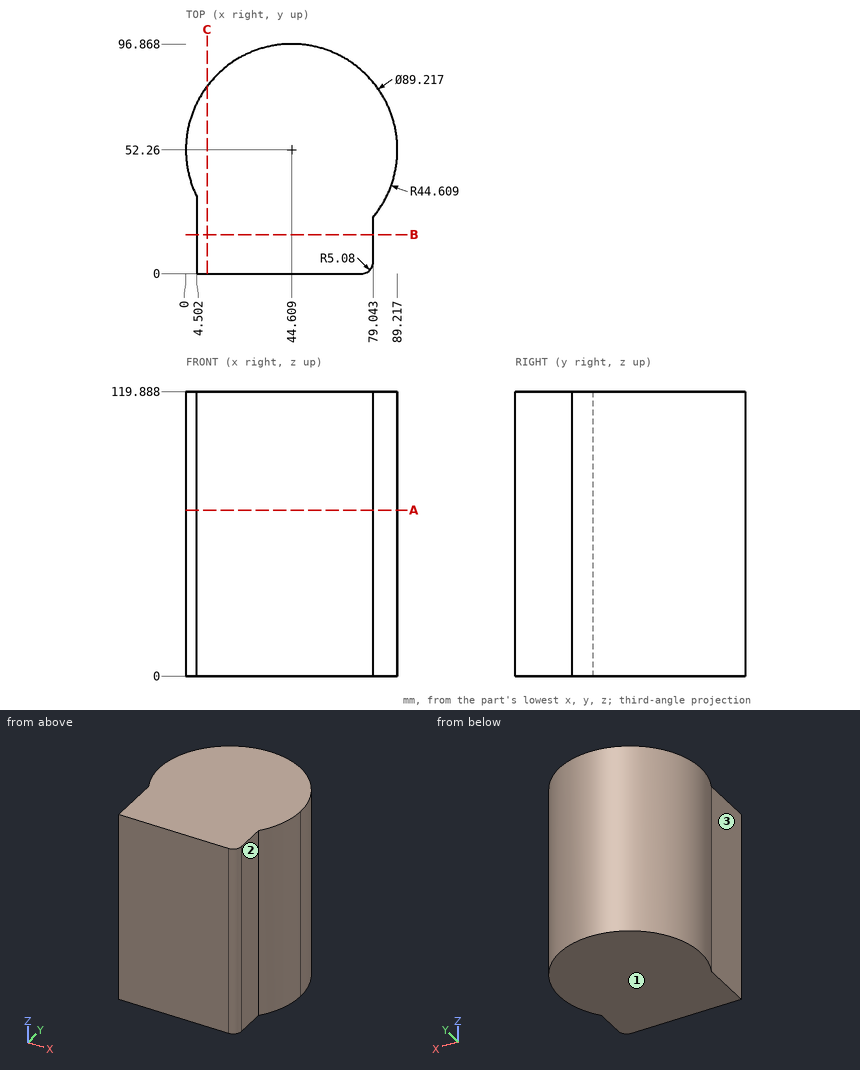
Input: dimensioned drawing with shaded views. Units: mm. Origin: part minimum x, y, z. A direction names the side the tool comes from. Give positions to 0.01 mm unless a question says otherwise; leave off trailing zeros. Order: outer loops, then holes, each group sorted by start corner. A loop starts at its lowest first (then second) coordinate and runs counter-clockwise, first axis right, second up. Notation, with made-up numbers: (-24, -6.5) -> (13, -6.5) arc R34 ccw to (13, 23.5) -> close; hole circle Ø4 at (2.5, -36.75). An arc over 180 degrees is marked (long way). Use a Markdown table: item, result.
1) Reachability of the marked faces 1, 2 and 3 from +Z, -Z, +X, -X, +Y, -Y: full face, straight path, thin tool, end or side. Return the list, or none.
Answer list:
| item | result |
|---|---|
| face 1 | -Z, +X, -X, +Y, -Y |
| face 2 | +Z, -Z, +X, -Y |
| face 3 | +Z, -Z, -X, -Y |
2) Section query B-B, the plane y = 16.5. Return the cut outline in (x, z).
Answer list:
| item | result |
|---|---|
| outline | (4.5, 0) -> (79.04, 0) -> (79.04, 119.89) -> (4.5, 119.89) -> close |
3) Section query C-C, the plane x = 9. Return the cut outline in (y, z), then the cut area to 3 significant figures.
Answer list:
| item | result |
|---|---|
| outline | (0, 0) -> (79.13, 0) -> (79.13, 119.89) -> (0, 119.89) -> close |
| area | 9,490 mm² |
4) Section query A-A, the plane z = 70. Return the cut outline in (x, y), then the cut area to 3 significant figures.
Answer list:
| item | result |
|---|---|
| outline | (4.5, 0) -> (73.96, 0) arc R5.08 ccw to (79.04, 5.08) -> (79.04, 23.9) arc R44.61 ccw to (89.22, 52.26) arc R44.61 ccw (long way) to (4.5, 32.73) -> close |
| area | 7,270 mm² |
5) Ray query, line 1 along X through (y, z) = (8, 75.5); line 2 along Y through (x, z) = (43, 100.5); line 3 along X through (y, z) = (53, 28). Return the intervals inside material, ascending. Write a range as [from, to].
Answer list:
| item | result |
|---|---|
| line 1 | [4.5, 79.04] |
| line 2 | [0, 96.84] |
| line 3 | [0.01, 89.21] |
6) Contact query for flat-ended pins moving along their axis: P1, Ø3, axis at x = 65.5, z = 70.5, coming from the +Y side; P2, Ø2, axis at x = 64, z = 87, coming from the +Y side; P3, Ø20.5, axis at y = 12.5, z = 43, coming from the +X side. Output: stop coordinate, or through.
Answer list:
| item | result |
|---|---|
| P1 | y = 92.43 |
| P2 | y = 92.9 |
| P3 | x = 79.04 |
